Work out the finished part from the listing and answer in its coordinate system (mm). Face numbers are marked on the shaded views. A direction names the side the tool comes from. Coordinates: 2 decimals unless noted, no trailing zeros. Loops run counter-clockwise (first coordinate to the right, second up) from the corner with the lowest first, then second, coordinate; pieces in that order, holes last. Notation, with made-up numbers: (-17, 70.5) - (34, 70.5) arc R9 ccw to (34, 76.5) - close; hole circle Ø11 at (68.5, 55.25). An arc over 180 degrees is marked (long way). Write each question's results on one line, items separated by ' | '. Start each with the question number.
1. A cutting plane is placed at D-D on y = 7. Determine the outline of the cut face in (x, z), then the cut area to 3 significant figures.
2. A cutting plane is placed at B-B on y = -7. Determine the outline of the cut face in (x, z).
3. A cutting plane is placed at A-A on x = 2.5. Determine the outline of the cut face in (y, z), then the cut area to 3 significant figures.
4. Each of these flat-tipped pins is pushed along its axis until it touches: P1, Ø1, axis at x = 1, z = 1.5, coming from the -Y side; P2, Ø0.8, axis at x = -6.5, z = 2.5, coming from the +Y side; P3, Ø0.6, axis at y = 9, z = 3.5, coming from the +X side. Where does it stop, or does it pass through?
5. Which of the six approach directions +Z, -Z, +X, -X, +Y, -Y give full straight-line access (tool end or side, diameter ignored) to the marked faces 4, 5 and 6?
6. A cutting plane is placed at C-C on x = 0. Determine the outline of the cut face in (y, z).
7. Find the intervals of material crossed by line 1 along Z through (x, y) = (2.45, 7); line 2 along Y through (x, z) = (0, 1.9); line 3 along Y through (x, z) = (-7.25, 4.25), in increasing order. Write a range as [from, to].
8. Determine the mould class of the marked faces 1, 2 and 3 for opening direction Y: released by +Y, released by -Y, zero draft, split by the parting line, or undercut.
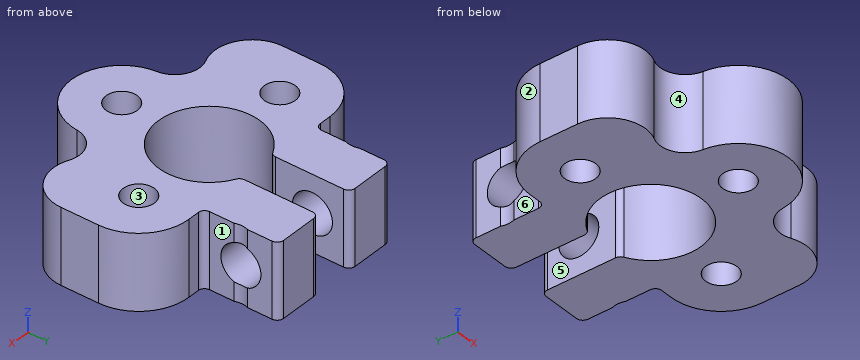
Autodesk Inventor part; units mm, degrees
ref_plane "YZ Plane" through (0, 0, 0) normal (1, 0, 0) x (0, 1, 0)
ref_plane "XZ Plane" through (0, 0, 0) normal (0, 1, 0) x (-1, 0, 0)
ref_plane "XY Plane" through (0, 0, 0) normal (0, 0, 1) x (1, 0, 0)
sketch "スケッチ1" plane through (0, 0, 0) normal (0, 0, 1) x (1, 0, 0)
  arc A0 (-1.55, 3.7417) -> (1.55, 3.7417) centre (0, 0) ccw
  circle A1 centre (-7, 0) radius 1.25
  circle A2 centre (7, 0) radius 1.25
  arc A3 (-7, 4) -> (-11, 0) centre (-7, 0) ccw
  arc A4 (11, 0) -> (7, 4) centre (7, 0) ccw
  line L0 (-1.55, 10) -> (-1.55, 3.7417)
  line L1 (1.55, 10) -> (1.55, 3.7417)
  circle A5 centre (0, -7) radius 1.25
  line L2 (1.55, 10) -> (5.55, 10)
  line L3 (5.55, 10) -> (5.55, 7.5385)
  line L4 (5.55, 4) -> (7, 4)
  line L5 (-1.55, 10) -> (-5.55, 10)
  line L6 (-5.55, 10) -> (-5.55, 7.5385)
  line L7 (-5.55, 4) -> (-7, 4)
  line L8 (-11, 0) -> (-11, -3)
  arc A6 (-11, -3) -> (-6.7837, -5.7424) centre (-8, -3) ccw
  arc A7 (1.55, 3.7417) -> (-1.55, 3.7417) centre (0, 0) ccw construction
  arc A8 (-3.9819, -7.3804) -> (3.9819, -7.3804) centre (0, -7) ccw
  arc A9 (-3.9819, -7.3804) -> (-6.7837, -5.7424) centre (-5.9728, -7.5706) ccw
  line L9 (11, 0) -> (11, -3)
  arc A10 (6.7837, -5.7424) -> (11, -3) centre (8, -3) ccw
  arc A11 (6.7837, -5.7424) -> (3.9819, -7.3804) centre (5.9728, -7.5706) ccw
  arc A12 (-5.55, 7.5385) -> (-5.55, 6.4615) centre (-6.95, 7) ccw construction
  arc A13 (5.55, 6.4615) -> (5.55, 7.5385) centre (6.95, 7) ccw construction
  arc A14 (-5.55, 6.4615) -> (-5.55, 7.5385) centre (-6.95, 7) ccw
  arc A15 (5.55, 7.5385) -> (5.55, 6.4615) centre (6.95, 7) ccw
  line L10 (5.55, 6.4615) -> (5.55, 4)
  line L11 (5.55, 7.5385) -> (5.55, 6.4615) construction
  line L12 (-5.55, 6.4615) -> (-5.55, 4)
  line L13 (-5.55, 7.5385) -> (-5.55, 6.4615) construction
  dimension "d0" = 8.1
  dimension "d1" = 2.5
  dimension "d2" = 2.5
  dimension "d4" = 7
  dimension "d5" = 7
  dimension "d6" = 2.5
  dimension "d7" = 7
  dimension "d8" = 6
  dimension "d9" = 4
  dimension "d10" = 3.1
  dimension "d11" = 4
  dimension "d12" = 4
  dimension "d13" = 1.55
  dimension "d14" = 3
  dimension "d15" = 3
  dimension "d16" = 4
  dimension "d17" = 4
  dimension "d18" = 3
  dimension "d19" = 3
  dimension "d20" = 2
  dimension "d21" = 2
  dimension "d22" = 3
  dimension "d23" = 3
  dimension "d24" = 1.4
  dimension "d25" = 1.4
  dimension "d26" = 3
  dimension "d27" = 3
extrude "押し出し1" add sketch "スケッチ1" along normal blind 6
sketch "スケッチ2" plane through (5.55, 4, 0) normal (1, 0, 0) x (0, 0, -1)
  circle A0 centre (-3, 3) radius 1.6
  line L0 (0, 6) -> (-6, 6)
  point P0 (0, -4)
  dimension "d30" = 3.2
  dimension "d31" = 3
  dimension "d32" = 3
extrude "押し出し2" cut sketch "スケッチ2" against normal through all
fillet "フィレット1" radius 0.5 8 edges at (-5.55, 10, 3) (-1.55, 10, 3) (1.55, 10, 3) (5.55, 10, 3) (5.55, 4, 3) (-5.55, 4, 3) (-1.55, 3.7417, 3) (1.55, 3.7417, 3)
properties part number "カップリング_軸8mm_2.5mm"
Values:
1) outline: (-5.45, 0) - (-1.55, 0) - (-1.55, 1.4) - (-5.45, 1.4) - close; (-5.45, 4.6) - (-1.55, 4.6) - (-1.55, 6) - (-5.45, 6) - close; (1.55, 0) - (5.45, 0) - (5.45, 1.4) - (1.55, 1.4) - close; (1.55, 4.6) - (5.45, 4.6) - (5.45, 6) - (1.55, 6) - close | area: 21.8 mm^2
2) outline: (-4.06, 0) - (-1.25, 0) - (-1.25, 6) - (-4.06, 6) - close; (1.25, 0) - (4.06, 0) - (4.06, 6) - (1.25, 6) - close
3) outline: (-10.12, 0) - (-3.19, 0) - (-3.19, 6) - (-10.12, 6) - close; (3.19, 0) - (10, 0) - (10, 6) - (3.19, 6) - close; hole circle Ø3.2 at (7, 3) | area: 74.5 mm^2
4) P1: y = -10.97 | P2: y = 4 | P3: x = 5.55
5) face 4: +Z, -Z, -Y | face 5: +Z, -Z, +Y | face 6: +Z, -Z, -X, +Y
6) outline: (-11, 0) - (-8.25, 0) - (-8.25, 6) - (-11, 6) - close; (-5.75, 0) - (-4.05, 0) - (-4.05, 6) - (-5.75, 6) - close
7) line 1: [0, 1.4], [4.6, 6] | line 2: [-11, -8.25], [-5.75, -4.05] | line 3: [-5.9, -1.22], [1.22, 3.99]
8) face 1: zero draft | face 2: released by +Y | face 3: undercut
